```python
from build123d import *

# Parameters (mm, degrees)
SKETCH1_W                    = 12.7
SKETCH1_H                    = 12.7
BOSS_EXTRUDE1_DEPTH          = 15.875
F_7_0_201_DIAMETER_HOLE1_D   = 5.1054
SKETCH5_W                    = 12.7
SKETCH5_H                    = 12.7
BOSS_EXTRUDE2_DEPTH          = 6.35
F_5_16_24_TAPPED_HOLE1_D     = 6.9088
F_5_16_24_TAPPED_HOLE1_DEPTH = 19.304
F_5_16_24_TAPPED_HOLE1_TIP   = 2.075612922
BOSS_EXTRUDE4_START          = 3.175
SKETCH9_W                    = 12.7
SKETCH9_H                    = 38.1
SKETCH9_R                    = 2.5527
BOSS_EXTRUDE4_DEPTH          = 3.175


with BuildPart() as part:
    # Sketch1 → Boss-Extrude1 (new, symmetric)
    with BuildSketch(Plane.XY):
        Rectangle(SKETCH1_W, SKETCH1_H)
    extrude(amount=BOSS_EXTRUDE1_DEPTH, both=True)

    # #7 (0.201) Diameter Hole1 (through all)
    with Locations(Plane(origin=(0, 6.35, 0), x_dir=(1, 0, 0), z_dir=(0, 1, 0))):
        with Locations((0, -3.175), (0, 9.525)):
            Hole(F_7_0_201_DIAMETER_HOLE1_D / 2)

    # Sketch5 → Boss-Extrude2 (add)
    with BuildSketch(Plane.XY.offset(15.875)):
        Rectangle(SKETCH5_W, SKETCH5_H)
    extrude(amount=BOSS_EXTRUDE2_DEPTH)

    # 5/16-24 Tapped Hole1
    with Locations(Plane.XY.offset(22.225)):
        with Locations((0, -2.54)):
            Hole(F_5_16_24_TAPPED_HOLE1_D / 2, depth=F_5_16_24_TAPPED_HOLE1_DEPTH)
            with Locations((0, 0, -(F_5_16_24_TAPPED_HOLE1_DEPTH + F_5_16_24_TAPPED_HOLE1_TIP / 2))):  # 118° drill point
                Cone(0, F_5_16_24_TAPPED_HOLE1_D / 2, F_5_16_24_TAPPED_HOLE1_TIP, mode=Mode.SUBTRACT)

    # Sketch9 → Boss-Extrude4 (add)
    with BuildSketch(Plane.XZ.offset(6.35).offset(BOSS_EXTRUDE4_START)):
        with Locations((0, 3.175)):
            Rectangle(SKETCH9_W, SKETCH9_H)
        with Locations(Location((0, 3.175, 0), (0, 0, 90))):
            Circle(SKETCH9_R, mode=Mode.SUBTRACT)
        with Locations(Location((0, -9.525, 0), (0, 0, 90))):
            Circle(SKETCH9_R, mode=Mode.SUBTRACT)
    extrude(amount=-BOSS_EXTRUDE4_DEPTH)


solid = part.part
```
Here's how the part is built. I have some questions about the finished solid (model axes, mm). A direction names the side the tool comes from. Round coordinates to 2 decimals unless told otherwise and drop trailing zeros. Order: outer loops, then holes, each group sorted by start corner. A loop starts at its lowest first (then second) coordinate and runs counter-clockwise, first axis right, second up. Notation, with made-up numbers: M 60.25,35.5 L 68.25,35.5 A13 ccw 68.25,53.5 Z; hole C 78.5,27 d7. An arc over 180 degrees is marked long. Use CSV: the item, a comma, the result in double quotes.
1) I want a section at A-A (x = 0). List the corners of the cut face in (y, z) for me (3 decimals), then the cut area to 3 significant figures.
Taken from the geometry:
outline,"M -9.525,-15.875 L 6.35,-15.875 L 6.35,-12.078 L -9.525,-12.078 Z; M -9.525,-6.972 L 6.35,-6.972 L 6.35,0.622 L -9.525,0.622 Z; M -9.525,5.728 L -5.994,5.728 L -5.994,22.225 L -9.525,22.225 Z; M 0.914,5.728 L 6.35,5.728 L 6.35,22.225 L 0.914,22.225 Z"
area,"329 mm^2"
2) I need wall thicknesses on line 1 along Z through (x, y) = (0, 1.75) (3 decimals); line 2 along Z through (x, y) = (-1.5, -8) (1 decimal); line 3 along Y through (x, z) = (0, 10.75) (3 decimals). Which ranges of each line are inside material? Lowest first, please. Write a range as [from, to].
Taken from the geometry:
line 1,"[-15.875, -12.078], [-6.972, 0.622], [5.728, 22.225]"
line 2,"[-15.9, -11.6], [-7.5, 1.1], [5.2, 22.2]"
line 3,"[-9.525, -5.994], [0.914, 6.35]"
3) If we mould it in two halves opening along Z, with no side actions, what happens to faces 1 (the flat face through (3, 0, 22.225)), 2 (the flat face through (3, 6.35, 3)), 3 (the cylindrical face through (-2.17, -1.7, 1.83))? For each: pulls with the +Z half, pulls with the -Z half, needs draft (parallel to the pull), parting line crosses it, or undercut.
Taken from the geometry:
face 1,"pulls with the +Z half"
face 2,"needs draft"
face 3,"undercut"
4) I want a section at B-B (z = 19.5). List the corners of the cut face in (x, y) for me (3 decimals), then the cut area to 3 significant figures.
Taken from the geometry:
outline,"M -6.35,-9.525 L 6.35,-9.525 L 6.35,6.35 L -6.35,6.35 Z; hole C 0,-2.54 d6.909"
area,"164 mm^2"
5) I'm going to push a flat-ended pin straight in: P1, Ø3, axis at x = 0, z = 3.175, coming from the -Y side. Where does the tip first touch, or does it pass through?
Taken from the geometry:
P1,"through"
6) On a 3-axis mill with a long thin cutter (end or side, diameter ignored), from which of +Z, -Z, +X, -X, +Y, -Y can I reach the whole of each face in a straight line? I mean faces 4 (the flat face through (3, -9.525, 3)), 5 (the conical face through (2.93, -2.571, 2.606)). Say none if no direction works.
Taken from the geometry:
face 4,"+Z, -Z, +X, -X, -Y"
face 5,"+Z"
7) I want a section at C-C (y = -2.54). List the corners of the cut face in (x, z) for me (3 decimals).
Taken from the geometry:
outline,"M -6.35,-15.875 L 6.35,-15.875 L 6.35,22.225 L 3.454,22.225 L 3.454,2.921 L 2.392,2.282 A2.553 cw -2.392,2.282 L -3.454,2.921 L -3.454,22.225 L -6.35,22.225 Z; hole C 0,-9.525 d5.105"
8) I want a section at D-D (z = 4). List the corners of the cut face in (x, y) for me (3 decimals).
Taken from the geometry:
outline,"M -6.35,-9.525 L -2.416,-9.525 L -2.416,-5.009 A3.454 cw -2.416,-0.071 L -2.416,6.35 L -6.35,6.35 Z; M 2.416,-9.525 L 6.35,-9.525 L 6.35,6.35 L 2.416,6.35 L 2.416,-0.071 A3.454 cw 2.416,-5.009 Z"
